Read the model definition and answer for the solid it produces. Units are mm, in the model's axes. Face numbers are marked on the shaded views. A direction names the side the tool comes from. Coordinates: 2 decimals unless noted, no trailing zeros. Write each loop counter-clockwise with the first axis right and the second up, starting at its lowest first coordinate (ties: lowest second). Pieces come first, ordered by that corner, then holes. Notation, with made-up numbers: (32, 38.5) -> (46, 38.5) arc R24 ccw to (46, 65.5) -> close; hole circle Ø8 at (25.25, -24.75). An arc over 180 degrees is marked (long way). One line per item, written item: value. Start each with the question number.
1. For a pull along Z with two mould halves and no side action, classify the marked faces 3, 4 and 5 as pulls with the +Z half, pulls with the -Z half, needs draft (parallel to the pull), parting line crosses it, or undercut.
2. Find section B-B, the plane x = -6.75. Write down the section's boundary in (y, z), and give its area (3 significant figures).
3. Find section A-A, the plane y = 2. Write down the section's boundary in (x, z), and give its area (3 significant figures).
4. Given P1, Ø3.5, axis at x = -11, z = -2, coming from the +Y side; P2, Ø1.3, axis at x = -7.5, z = -1.5, coming from the -Y side, each flat-ended and moving along its own axis, determine where each tip first touches the part or whether it passes through.
5. Consider line 1 along Z through (x, y) = (-8.5, -46); line 2 along X through (y, z) = (-79, 20); line 3 along X through (y, z) = (-21, 3). Determine where each line is inside the solid, lowest interval first.
6. For the marked faces 1 and 2, determine the directions among +Z, -Z, +X, -X, +Y, -Y from which every point of the face is accessible in a straight line to the end or side of a thin tool.
```python
from build123d import *

# Parameters (mm, degrees)
EXTRUDE001_DEPTH      = 170
EXTRUDE001_DEPTH_BACK = 25
EXTRUDE_DEPTH         = 145
FILLET_R              = 1
FILLET001_R           = 1


with BuildPart() as extrude001:
    # Sketch001 → Extrude001 (new body, two sides)
    with BuildSketch(Plane.XZ) as extrude001_sk:
        with BuildLine():
            Line((-18.336975, -4.599435), (-9.5, 44.269675))
            ThreePointArc((-9.5, 44.269675), (-9.634289, 44.777491), (-10.110105, 45))
            Line((-10.110105, 45), (-21.031197, 45))
            ThreePointArc((-21.031197, 45), (-22.069798, 44.569798), (-22.5, 43.531197))
            Line((-22.5, 43.531197), (-22.5, -4.084046))
            ThreePointArc((-22.5, -4.084046), (-22.231723, -4.731723), (-21.584046, -5))
            Line((-21.584046, -5), (-18.81647, -5))
            ThreePointArc((-18.81647, -5), (-18.504073, -4.886682), (-18.336975, -4.599435))
        make_face()
    extrude(amount=EXTRUDE001_DEPTH)
    extrude(extrude001_sk.sketch, amount=-EXTRUDE001_DEPTH_BACK)


with BuildPart() as fillet001:
    # Sketch → Extrude (new body)
    with BuildSketch(Plane.XZ):
        with BuildLine():
            Line((-4.690516, 0), (-14.717051, 0))
            ThreePointArc((-17.006162, 2.739987), (-16.502237, 0.834781), (-14.717051, 0))
            Line((-17.006162, 2.739987), (-9.5, 44.265571))
            ThreePointArc((-9.5, 44.265571), (-9.635072, 44.776244), (-10.113575, 45))
            Line((-10.113575, 45), (-21.031197, 45))
            ThreePointArc((-21.031197, 45), (-22.069798, 44.569798), (-22.5, 43.531197))
            Line((-22.5, 43.531197), (-22.5, -4.084046))
            ThreePointArc((-22.5, -4.084046), (-22.231723, -4.731723), (-21.584046, -5))
            Line((-21.584046, -5), (-4.064727, -5))
            ThreePointArc((-4.064727, -5), (-2.958298, -4.541702), (-2.5, -3.435273))
            Line((-2.5, -3.435273), (-2.5, -2.190516))
            ThreePointArc((-2.5, -2.190516), (-3.141587, -0.641587), (-4.690516, 0))
        make_face()
    extrude(amount=EXTRUDE_DEPTH)

    # Fillet
    fillet_edges = [fillet001.edges().sort_by_distance(p)[0] for p in [
        (-9.703783, 0, 0),
        (-9.703783, -145, 0),
        (-16.502237, 0, 0.834781),
        (-16.502237, -145, 0.834781),
        (-12.824386, 0, -5),
        (-12.824386, -145, -5),
        (-2.958298, 0, -4.541702),
        (-2.958298, -145, -4.541702),
        (-2.5, 0, -2.812895),
        (-2.5, -145, -2.812895),
        (-3.141587, 0, -0.641587),
        (-3.141587, -145, -0.641587),
    ]]
    fillet(fillet_edges, radius=FILLET_R)

    # Fusion: union Extrude001
    add(extrude001.part)

    # Fillet001
    fillet001_edges = [fillet001.edges().sort_by_distance(p)[0] for p in [
        (-13.918487, 25, 19.83512),
        (-13.918487, -170, 19.83512),
        (-9.634289, 25, 44.777491),
        (-15.570651, 25, 45),
        (-22.069798, 25, 44.569798),
        (-22.5, 25, 19.723576),
        (-22.231723, 25, -4.731723),
        (-20.200258, 25, -5),
        (-18.504073, 25, -4.886682),
        (-9.634289, -170, 44.777491),
        (-15.570651, -170, 45),
        (-22.069798, -170, 44.569798),
        (-22.5, -170, 19.723575),
        (-22.231723, -170, -4.731723),
        (-20.200258, -170, -5),
        (-18.504073, -170, -4.886682),
    ]]
    fillet(fillet001_edges, radius=FILLET001_R)


solid = fillet001.part
```
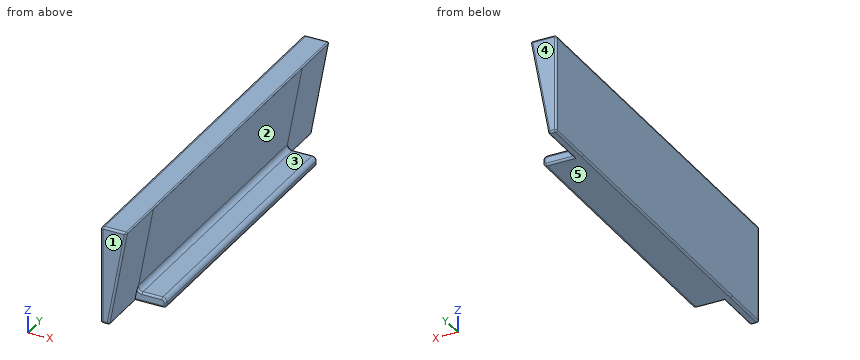
Answer block:
1. face 3: undercut
1. face 4: needs draft
1. face 5: pulls with the -Z half
2. outline: (-145, -4) arc R1 ccw to (-144, -5) -> (-1, -5) arc R1 ccw to (0, -4) -> (0, -1) arc R1 ccw to (-1, 0) -> (-144, 0) arc R1 ccw to (-145, -1) -> close
2. area: 724 mm2
3. outline: (-22.5, -4.08) arc R0.92 ccw to (-21.58, -5) -> (-18.82, -5) arc R0.49 ccw to (-18.34, -4.6) -> (-9.5, 44.27) arc R0.62 ccw to (-10.11, 45) -> (-21.03, 45) arc R1.47 ccw to (-22.5, 43.53) -> close
3. area: 430 mm2
4. P1: stops at y = 0
4. P2: stops at y = -145
5. line 1: z = -5 to 0
5. line 2: x = -22.5 to -13.89
5. line 3: x = -22.5 to -16.96
6. face 1: +Z, -Z, +X, -X, -Y
6. face 2: +X, +Y, -Y
